Autodesk Fusion 360 part; units mm, degrees
sketch "Sketch1" plane through (0, 0, 0) normal (0, 0, 1) x (1, 0, 0)
  line L0 (0, 0) -> (41, 0)
  line L1 (41, 0) -> (41, 35)
  line L2 (41, 35) -> (0, 35)
  line L3 (0, 35) -> (0, 0)
  line L4 (0, 17.5) -> (41, 17.5) construction
  circle A0 centre (4.8, 24.5) radius 2.75
  circle A1 centre (4.8, 10.5) radius 2.75
  line L5 (4.8, 24.5) -> (4.8, 10.5) construction
  line L6 (2.05, 10.5) -> (4.8, 10.5) construction
  line L7 (41, 42.475) -> (70, 42.475)
  line L8 (70, 42.475) -> (70, 2.475)
  line L9 (70, 2.475) -> (41, 2.475)
  line L10 (41, 2.475) -> (41, 0)
  line L11 (48.5, 34.45) -> (48.5, 10.5) construction
  circle A2 centre (48.5, 34.45) radius 2.75
  circle A3 centre (48.5, 10.5) radius 2.75 construction
  line L12 (70, 22.475) -> (48.5, 22.475) construction
  line L13 (41, 42.475) -> (41, 35)
  line L14 (0, 35) -> (0, 42.475)
  line L15 (0, 42.475) -> (41, 42.475)
  line L16 (62.8, 34.45) -> (62.8, 10.5) construction
  circle A4 centre (62.8, 34.45) radius 2.75 construction
  circle A5 centre (62.8, 10.5) radius 2.75
  line L17 (48.5, 34.45) -> (62.8, 34.45) construction
  line L18 (48.5, 10.5) -> (62.8, 10.5) construction
  line L19 (35.4, 24.5) -> (35.4, 10.5) construction
  circle A6 centre (35.4, 24.5) radius 2.75
  circle A7 centre (35.4, 10.5) radius 2.75
  point P0 (2.05, 10.5)
  dimension "d1" = 41
  dimension "d2" = 35
  dimension "d3" = 14
  dimension "d7" = 40
  dimension "d8" = 7.5
  dimension "d9" = 5.5
  dimension "d12" = 23.95
  dimension "d13" = 4.8
  dimension "d14" = 5.5
  dimension "d20" = 14.3
  dimension "d21" = 30.6
  dimension "d22" = 29
extrude "Extrude1" add sketch "Sketch1" along normal blind 6
extrude "Extrude2" cut sketch "Sketch1" along normal blind 2.1 from surface at 2 contours L0 L1 L2 L3 L10
equation "d3 = ( ( 9 + 19 ) / 2 ) * 1 mm"
equation "d8 = ( ( 4 + 11 ) / 2 ) * 1 mm"
equation "d12 = ( ( 17.5 + 30.4 ) / 2 ) * 1 mm"
equation "d15 = 2 mm + 2 mm + 2 mm"
equation "d20 = ( 18.3 mm - 4 mm )"
equation "d21 = ( ( 25.6 + 35.6 ) / 2 ) * 1 mm"
Verification items for the finished model (mm, model axes). A direction names the side the tool comes from. Give positions to 0.01 mm unless a question says otherwise; leave off trailing zeros. Write each loop counter-clockwise with the first axis right and the second up, starting at its lowest first coordinate (ties: lowest second). Pieces come first, ordered by that corner, then holes. Notation, with made-up numbers: (86, 49) -> (131, 49) arc R16 cw to (131, 77) -> close; hole circle Ø8 at (39, 41.25). An arc over 180 degrees is marked (long way). Use CSV: the item, a comma, the result in double quotes.
(1) Set-up check for faces 1 (the cylindrical face through (2.053, 10.379, 5.037)), 2 (the flat face through (56, 2.475, 3)), 3 (the flat face through (20, 18, 2)): record each of +Z, -Z, +X, -X, +Y, -Y from which the full face is reachable in a straight line by a thin tool's end or side.
Derived:
face 1,"+Z, -Z"
face 2,"+Z, -Z, +X, -Y"
face 3,"-X, -Y"
(2) Sectioned sample at A-A (x = 4.8). Record the cut outline in (y, z) (3 decimals), plus the area to 3 significant figures.
Derived:
outline,"(0, 0) -> (7.75, 0) -> (7.75, 2) -> (0, 2) -> close; (0, 4.1) -> (7.75, 4.1) -> (7.75, 6) -> (0, 6) -> close; (13.25, 0) -> (21.75, 0) -> (21.75, 2) -> (13.25, 2) -> close; (13.25, 4.1) -> (21.75, 4.1) -> (21.75, 6) -> (13.25, 6) -> close; (27.25, 0) -> (42.475, 0) -> (42.475, 6) -> (27.25, 6) -> (27.25, 4.1) -> (35, 4.1) -> (35, 2) -> (27.25, 2) -> close"
area,"138 mm^2"
(3) Sectioned sample at D-D (x = 48.5). Record the cut outline in (y, z) (3 decimals).
Derived:
outline,"(2.475, 0) -> (31.7, 0) -> (31.7, 6) -> (2.475, 6) -> close; (37.2, 0) -> (42.475, 0) -> (42.475, 6) -> (37.2, 6) -> close"
(4) Go/stop test with flat-tipped pins: pin 1 (0.6 mm diameter, centred on y = 13, z = 3.5, fed in from -X); pin 2 (3 mm diameter, centred on x = 53.5, z = 4.5, fed in from -Y) (3 decimals); pin 3 (0.6 mm diameter, centred on y = 0.5, z = 1, fed in from +X). Record where each tip stops, or that it passes through.
Derived:
pin 1,"stops at x = 41"
pin 2,"stops at y = 2.475"
pin 3,"stops at x = 41"
(5) Material ranges on L1, parallel to Y at x = 4.8, z = 4.9 (3 decimals); L2, parallel to Z at x = 28, y = 22.5; L3, parallel to Y at x = 62.8, z = 2.2 (3 decimals), recorded low to high.
Derived:
L1,"y = 0 to 7.75, 13.25 to 21.75, 27.25 to 42.475"
L2,"z = 0 to 2, 4.1 to 6"
L3,"y = 2.475 to 7.75, 13.25 to 42.475"
(6) Sectioned sample at C-C (y = 24.5). Record the cut outline in (x, z), plus the area to 3 significant figures.
Derived:
outline,"(0, 0) -> (2.05, 0) -> (2.05, 2) -> (0, 2) -> close; (0, 4.1) -> (2.05, 4.1) -> (2.05, 6) -> (0, 6) -> close; (7.55, 0) -> (32.65, 0) -> (32.65, 2) -> (7.55, 2) -> close; (7.55, 4.1) -> (32.65, 4.1) -> (32.65, 6) -> (7.55, 6) -> close; (38.15, 0) -> (70, 0) -> (70, 6) -> (38.15, 6) -> (38.15, 4.1) -> (41, 4.1) -> (41, 2) -> (38.15, 2) -> close"
area,"291 mm^2"
(7) Release check for a two-part mould opening along Y. For faces 4 (the flat face through (41, 19, 3)), 5 (the flat face through (20, 0, 5)), 6 (the cylindrical face through (35.042, 21.773, 0.986)), 7 (the cylindrical face through (4.442, 21.773, 0.986)) record: +Y half, -Y half, draft (parallel to the pull), parting line (faces both ways), or undercut.
Derived:
face 4,"draft"
face 5,"-Y half"
face 6,"undercut"
face 7,"undercut"
(8) Sectioned sample at B-B (z = 3.2). Record the cut outline in (x, y) (3 decimals).
Derived:
outline,"(0, 35) -> (41, 35) -> (41, 2.475) -> (70, 2.475) -> (70, 42.475) -> (0, 42.475) -> close; hole circle Ø5.5 at (48.5, 34.45); hole circle Ø5.5 at (62.8, 10.5)"
